Check sheet for the modelled part. Datum: model origin and axes. Units: mm. Face numbers are marked on the shaded views. A direction names the side the tool comes from. Coordinates: 2 decimals unless noted, no trailing zeros. Order: outer loops, then holes, each group sorted by start corner. A loop starts at its lowest first (then second) coordinate and runs counter-clockwise, first axis right, second up.
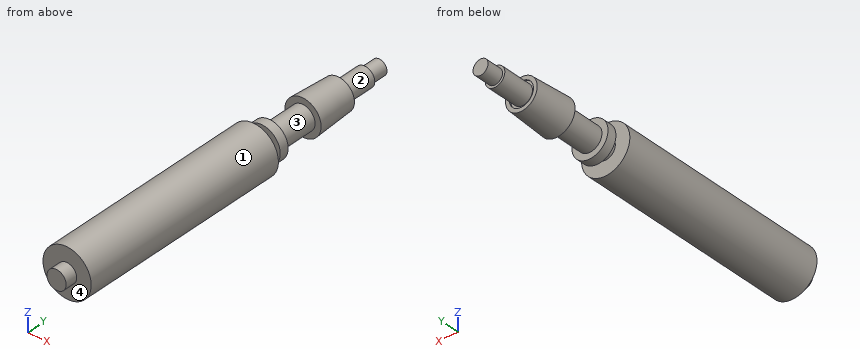
from build123d import *


with BuildPart() as part:
    # Çizim1 → Döndür1 (revolve)
    with BuildSketch(Plane.XY, mode=Mode.PRIVATE) as d_nd_r1_sk:
        Polygon((0, 0), (5, 0), (5, -11), (6.5, -11), (6.5, -32), (8, -32), (8, -31), (10.5, -31), (12, -58), (8, -58), (8, -83), (12, -83), (12, -89), (6.365949077, -89), (6.365949077, -95), (16, -95), (16, -237), (6.365949077, -237), (6.365949077, -245), (0, -245), align=None)
    revolve(d_nd_r1_sk.sketch.rotate(Axis((0, 0, 0), (0, -1, 0)), 90), axis=Axis((0, 0, 0), (0, -1, 0)))


solid = part.part
(1) Tool access check on the marked faces 1, 2, 3 and 4. Record the directions out of +Z, -Z, +X, -X, +Y, -Y that give a thin tool (end or side, any length) a straight path to the whole face; none if there is none.
Filled in:
face 1: +Y, -Y
face 2: +Y
face 3: none
face 4: -Y
(2) Cross-section at A-A (y = -18.5). Enter the section's corners in (x, z), and give its area (3 significant figures).
Filled in:
outline: circle Ø13 at (0, 0)
area: 133 mm2
(3) Thickness scan on probe 1 along X at (y, z) = (-31.6, 0); probe 2 along Y at (x, z) = (-7.5, -7); probe 3 along Y at (x, z) = (-6, -5). Record the ranges inside material, lowest first.
Filled in:
probe 1: x = -10.53 to -8, -6.5 to 6.5, 8 to 10.53
probe 2: y = -237 to -95, -89 to -83, -58 to -31
probe 3: y = -237 to -95, -89 to -32
(4) Go/stop test with flat-tipped pins: P1, Ø10, axis at y = -68, z = -2, coming from the +X side; P2, Ø4, axis at x = -10.5, z = -3, coming from the +Y side; P3, Ø8, axis at y = -46.5, z = -12, coming from the +X side; P4, Ø16, axis at x = -1, z = -8, coming from the -Y side. Record where each tip stops, or that it passes through.
Filled in:
P1: stops at x = 8
P2: stops at y = -31
P3: stops at x = 8.08
P4: stops at y = -245
(5) Cross-section at B-B (y = -153.5). Enter the section's corners in (x, z).
Filled in:
outline: circle Ø32 at (0, 0)
